Build history of the part. All positions in model axes, mm. A direction names the side the tool comes from. Coordinates: 2 decimals unless noted, no trailing zeros. Loops run counter-clockwise (first coordinate to the right, second up) from the corner with the lowest first, then second, coordinate; pieces in that order, holes last.
Item 1: Cut at C-C (z = 25). List the corners of the cut face in (x, y).
Item 2: 3-axis set-ups, long thin cutter, end or side, ignore diameter. For faces 4 (the face through (-6, 20, 19)), 5 (the face through (-6.35, 18, 0)), 6 (the face through (6.35, 18, 0)), 7 (the face through (6, 20, 19)), 8 (the face through (0, 24, 14.989)): which of +Z, -Z, +X, -X, +Y, -Y reach the whole face in a straight line?
Item 3: Cut at B-B (y = 142.5). List the corners of the cut face in (x, z).
Item 4: Cut at A-A (x = 25). List the corners of the cut face in (y, z), and give its area (3 significant figures).
Item 5: Mould opens along Z. For faces 1 (the face through (5, 149, 13)), 2 (the face through (-17.57, 6.26, -20.09)), 3 (the face through (-3, 133, 0)) say: released by +Z, released by -Z, zero draft, split by the parting line, or undercut.
Item 6: Flat gauge pins, fed straight in: pin 1 (8 mm diameter, centred on y = 92, z = -14, fed in from +X); pin 2 (3.5 mm diameter, centred on x = 4.5, z = 20.5, fed in from +Y); pin 3 (12 mm diameter, centred on x = -14.5, y = 88.5, fed in from +Z); pin 4 (6.5 mm diameter, centred on x = -17.68, z = -17.68, fed in from +Y). Where does each tip first touch, or does it go through?
Item 7: Drill centre lines: line 1 along X through (y, z) = (4.25, 0); line 2 along Y through (x, z) = (4.85, 30); line 3 along Z through (x, y) = (-6.6, 25). Where is each one in solid material? Low to high.
Item 8: Cut at D-D (y = 25). List the corners of the cut face in (x, z).
from build123d import *

# Parameters (mm, degrees)
SKETCH1_W               = 65
SKETCH1_H               = 65
BOSS_EXTRUDE1_DEPTH     = 12.7
SKETCH2_R               = 2
BOSS_EXTRUDE2_DEPTH     = 6.35
FILLET1_R               = 2.5
CUT_EXTRUDE2_DEPTH      = 157.883714897
CUT_EXTRUDE2_DEPTH_BACK = 12.7
SKETCH3_R               = 2.413
SKETCH4_R               = 2.032
BOSS_EXTRUDE4_DEPTH     = 7.6
CUT_EXTRUDE3_DEPTH      = 12.45
SKETCH6_W               = 6
SKETCH6_H               = 30
SKETCH6_H_2             = 5
CUT_EXTRUDE4_DEPTH      = 161.662690131


with BuildPart() as part:
    # Sketch1 → Boss-Extrude1 (new body)
    with BuildSketch(Plane(origin=(0, 0, 0), x_dir=(1, 0, 0), z_dir=(0, 1, 0))):
        Rectangle(SKETCH1_W, SKETCH1_H)
    extrude(amount=BOSS_EXTRUDE1_DEPTH)

    # Sketch2 → Boss-Extrude2 (add, symmetric)
    with BuildSketch(Plane(origin=(0, 0, 0), x_dir=(0, 0, -1), z_dir=(1, 0, 0))):
        with BuildLine():
            Line((-15, 0), (15, 0))
            Line((15, 0), (15, 145))
            ThreePointArc((15, 145), (13.535533906, 148.535533906), (10, 150))
            Line((10, 150), (-10, 150))
            ThreePointArc((-10, 150), (-13.535533906, 148.535533906), (-15, 145))
            Line((-15, 145), (-15, 0))
        make_face()
        with Locations((0, 142.5)):
            Circle(SKETCH2_R, mode=Mode.SUBTRACT)
    extrude(amount=BOSS_EXTRUDE2_DEPTH, both=True)

    # Fillet1
    fillet1_edges = [part.edges().sort_by_distance(p)[0] for p in [
        (32.5, 12.7, 0),
        (0, 12.7, -32.5),
        (-6.35, 12.7, 0),
        (0, 12.7, 15),
        (0, 12.7, -15),
        (6.35, 12.7, 0),
        (-32.5, 12.7, 0),
        (-32.5, 6.35, -32.5),
        (32.5, 6.35, -32.5),
        (32.5, 6.35, 32.5),
        (-32.5, 6.35, 32.5),
        (0, 12.7, 32.5),
    ]]
    fillet(fillet1_edges, radius=FILLET1_R)

    # Sketch3 → Cut-Extrude2 (cut, two sides: drawn at the far end of the back side and taken through both)
    with BuildSketch(Plane(origin=(0, 0, 0), x_dir=(1, 0, 0), z_dir=(0, 1, 0)).offset(-CUT_EXTRUDE2_DEPTH_BACK)):
        with Locations(Location((17.67766953, -17.67766953, 0), (0, 0, 270))):
            Circle(SKETCH3_R)
        with Locations(Location((25, 0, 0), (0, 0, 270))):
            Circle(SKETCH3_R)
        with Locations(Location((17.67766953, 17.67766953, 0), (0, 0, 270))):
            Circle(SKETCH3_R)
        with Locations(Location((0, 25, 0), (0, 0, 270))):
            Circle(SKETCH3_R)
        with Locations(Location((-17.67766953, 17.67766953, 0), (0, 0, 270))):
            Circle(SKETCH3_R)
        with Locations(Location((-25, 0, 0), (0, 0, 270))):
            Circle(SKETCH3_R)
        with Locations(Location((-17.67766953, -17.67766953, 0), (0, 0, 270))):
            Circle(SKETCH3_R)
        with Locations(Location((0, -25, 0), (0, 0, 270))):
            Circle(SKETCH3_R)
    extrude(amount=CUT_EXTRUDE2_DEPTH + CUT_EXTRUDE2_DEPTH_BACK, mode=Mode.SUBTRACT)

    # Sketch4 → Boss-Extrude4 (add, symmetric)
    with BuildSketch(Plane(origin=(0, 0, 0), x_dir=(0, 0, -1), z_dir=(1, 0, 0))):
        with BuildLine():
            Line((15, 20), (-32.5, 20))
            ThreePointArc((-32.5, 20), (-34.267766953, 20.732233047), (-35, 22.5))
            Line((-35, 22.5), (-35, 27.5))
            ThreePointArc((-35, 27.5), (-34.267766953, 29.267766953), (-32.5, 30))
            Line((-32.5, 30), (15, 30))
            Line((15, 30), (15, 20))
        make_face()
        with Locations(Location((-30, 25, 0), (0, 0, 180))):
            Circle(SKETCH4_R, mode=Mode.SUBTRACT)
    extrude(amount=BOSS_EXTRUDE4_DEPTH, both=True)

    # Sketch5 → Cut-Extrude3 (cut)
    with BuildSketch(Plane(origin=(0, 30, 0), x_dir=(1, 0, 0), z_dir=(0, 1, 0))):
        Polygon((-3.070505438, -14.989300838), (-3.070505438, -44.384490964), (3.070505438, -44.384490964), (2.929494562, -14.989300838), align=None)
    extrude(amount=-CUT_EXTRUDE3_DEPTH, mode=Mode.SUBTRACT)

    # Sketch6 → Cut-Extrude4 (cut, through all)
    with BuildSketch(Plane.XY.offset(15)):
        with Locations((0, 130)):
            Rectangle(SKETCH6_W, SKETCH6_H)
        with Locations((0, 147.5)):
            Rectangle(SKETCH6_W, SKETCH6_H_2)
    extrude(amount=-CUT_EXTRUDE4_DEPTH, mode=Mode.SUBTRACT)


solid = part.part
Filled sheet:
1. outline: (-32.5, 0) - (-2.41, 0) - (-2.41, 12.7) - (-30, 12.7) arc R2.5 ccw to (-32.5, 10.2) - close; (-7.6, 20) - (-3.07, 20) - (-3.07, 30) - (-7.6, 30) - close; (2.41, 0) - (32.5, 0) - (32.5, 10.2) arc R2.5 ccw to (30, 12.7) - (2.41, 12.7) - close; (2.98, 20) - (7.6, 20) - (7.6, 30) - (2.98, 30) - close
2. face 4: +Z, -X
2. face 5: +Z, -Z, -X
2. face 6: +Z, -Z, +X
2. face 7: +Z, +X
2. face 8: +Z, +Y
3. outline: (-6.35, -15) - (-3, -15) - (-3, -2) - (-6.35, -2) - close; (-6.35, 2) - (-3, 2) - (-3, 15) - (-6.35, 15) - close; (3, -15) - (6.35, -15) - (6.35, -2) - (3, -2) - close; (3, 2) - (6.35, 2) - (6.35, 15) - (3, 15) - close
4. outline: (0, -32.5) - (10.2, -32.5) arc R2.5 ccw to (12.7, -30) - (12.7, -2.41) - (0, -2.41) - close; (0, 2.41) - (12.7, 2.41) - (12.7, 30) arc R2.5 ccw to (10.2, 32.5) - (0, 32.5) - close
4. area: 762 mm2
5. face 1: released by +Z
5. face 2: undercut
5. face 3: zero draft
6. pin 1: stops at x = 6.35
6. pin 2: stops at y = 30
6. pin 3: passes through
6. pin 4: stops at y = 12.7
7. line 1: x = -32.5 to -27.41, -22.59 to 22.59, 27.41 to 32.5
7. line 2: y = 0 to 12.7, 20 to 22.97, 27.03 to 30
7. line 3: z = -15 to 27.97, 32.03 to 35
8. outline: (-7.6, -15) - (7.6, -15) - (7.6, 27.97) - (2.99, 27.97) - (2.93, 14.99) - (-3.07, 14.99) - (-3.07, 27.97) - (-7.6, 27.97) - close; (-7.6, 32.03) - (-3.07, 32.03) - (-3.07, 35) - (-7.6, 35) - close; (3.01, 32.03) - (7.6, 32.03) - (7.6, 35) - (3.03, 35) - close
